from build123d import *

# Parameters (mm, degrees)
BOSS_EXTRUDE1_DEPTH = 135
SKETCH3_R           = 3.25
CUT_EXTRUDE2_DEPTH  = 10
SKETCH6_W           = 11
SKETCH6_H           = 36
CUT_EXTRUDE3_DEPTH  = 40
SKETCH7_W           = 55
SKETCH7_H           = 16.435142828
BOSS_EXTRUDE2_DEPTH = 35
CUT_EXTRUDE4_DEPTH  = 20
CUT_EXTRUDE5_DEPTH  = 20
SKETCH12_R          = 3.5
CUT_EXTRUDE6_DEPTH  = 10
CUT_EXTRUDE7_DEPTH  = 120
SKETCH14_W          = 10
SKETCH14_H          = 112.990035736
BOSS_EXTRUDE3_DEPTH = 9


with BuildPart() as part:
    # Sketch2 → Boss-Extrude1 (new body)
    with BuildSketch(Plane.XY):
        with BuildLine():
            Line((-7.403081865, 56.261800555), (-7.403081865, -78.738199445))
            ThreePointArc((-7.403081865, -78.738199445), (0.096918135, -86.238199445), (7.596918135, -78.738199445))
            Line((7.596918135, -78.738199445), (7.596918135, 56.261800555))
            ThreePointArc((7.596918135, 56.261800555), (0.096918135, 63.761800555), (-7.403081865, 56.261800555))
        make_face()
    extrude(amount=BOSS_EXTRUDE1_DEPTH)

    # Sketch3 → Cut-Extrude2 (cut)
    with BuildSketch(Plane(origin=(0, 0, 0), x_dir=(-1, 0, 0), z_dir=(0, 0, -1))):
        with Locations((-0.096918135, 54.761800555)):
            Circle(SKETCH3_R)
    extrude(amount=-CUT_EXTRUDE2_DEPTH, mode=Mode.SUBTRACT)

    # Sketch6 → Cut-Extrude3 (cut)
    with BuildSketch(Plane(origin=(0, 0, 0), x_dir=(-1, 0, 0), z_dir=(0, 0, -1))):
        with Locations((-0.096918135, -48.578199445)):
            Rectangle(SKETCH6_W, SKETCH6_H)
    extrude(amount=-CUT_EXTRUDE3_DEPTH, mode=Mode.SUBTRACT)

    # Sketch7 → Boss-Extrude2 (add)
    with BuildSketch(Plane.ZY.offset(7.403081865)):
        with Locations((67.5, -49.750557846)):
            Rectangle(SKETCH7_W, SKETCH7_H)
    extrude(amount=BOSS_EXTRUDE2_DEPTH)

    # Sketch10 → Cut-Extrude4 (cut)
    with BuildSketch(Plane(origin=(0, -41.532986432, 0), x_dir=(1, 0, 0), z_dir=(0, 1, 0))):
        with BuildLine():
            Line((-7.403081865, -40), (-42.403081865, -40))
            Line((-42.403081865, -40), (-42.403081865, -95))
            Line((-42.403081865, -95), (-7.403081865, -95))
            ThreePointArc((-7.403081865, -95), (-33.21161021, -67.5), (-7.403081865, -40))
        make_face()
    extrude(amount=-CUT_EXTRUDE4_DEPTH, mode=Mode.SUBTRACT)

    # Sketch11 → Cut-Extrude5 (cut)
    with BuildSketch(Plane(origin=(0, -41.532986432, 0), x_dir=(1, 0, 0), z_dir=(0, 1, 0))):
        with BuildLine():
            Line((-7.569996139, -52.041059143), (-7.569996139, -82.958940857))
            ThreePointArc((-7.569996139, -82.958940857), (-23.028936996, -67.5), (-7.569996139, -52.041059143))
        make_face()
    extrude(amount=-CUT_EXTRUDE5_DEPTH, mode=Mode.SUBTRACT)

    # Sketch12 → Cut-Extrude6 (cut)
    with BuildSketch(Plane.XY.offset(135)):
        with Locations((0.096918135, 54.761800555)):
            Circle(SKETCH12_R)
    extrude(amount=-CUT_EXTRUDE6_DEPTH, mode=Mode.SUBTRACT)

    # Sketch13 → Cut-Extrude7 (cut)
    with BuildSketch(Plane.XY.offset(135)):
        Polygon((4.403081865, 46.751836291), (-4.403081865, 46.751836291), (-4.403081865, -46.751836291), (-4.403081865, -66.238199445), (4.403081865, -66.238199445), (4.403081865, -46.751836291), align=None)
    extrude(amount=-CUT_EXTRUDE7_DEPTH, mode=Mode.SUBTRACT)

    # Sketch14 → Boss-Extrude3 (add)
    with BuildSketch(Plane.ZY.offset(-4.403081865)):
        with Locations((130, -9.743181577)):
            Rectangle(SKETCH14_W, SKETCH14_H)
    extrude(amount=BOSS_EXTRUDE3_DEPTH)


solid = part.part
Input: part model. Units: mm. Frame: model coordinates. A direction names the side the tool comes from. Give positions to 0.01 mm unless a question says otherwise; leave off trailing zeros. Loops run counter-clockwise (first coordinate to the right, second up) from the corner with the lowest first, then second, coordinate; pieces in that order, holes last. Notation, with made-up numbers: M 1.5,8 L 33.5,8 A30 ccw 33.5,33 Z; hole C -10,27.25 d6. An arc over 180 degrees is marked long. Use CSV: the item, a comma, the result in double quotes.
(1) Material intervals for L1, parallel to X at y = -18.5, z = 112; L2, parallel to Z at x = 0.5, y = -15; L3, parallel to Y at x = -4, z = 61.5, sorted ascending. Write a range as [from, to].
Outcome:
L1,"x = [-7.4, -4.4], [4.4, 7.6]"
L2,"z = [0, 15], [125, 135]"
L3,"y = [-85.02, -66.24], [46.75, 62.54]"
(2) Section A-A, the plane z = 67.5. Return loops of the section in (x, y), plus the area to 3 significant figures.
Outcome:
outline,"M -33.21,-57.97 L -23.03,-57.97 L -23.03,-41.53 L -33.21,-41.53 Z; M -7.57,-57.97 L -7.4,-57.97 L -7.4,-78.74 A7.5 ccw 7.6,-78.74 L 7.6,56.26 A7.5 ccw -7.4,56.26 L -7.4,-41.53 L -7.57,-41.53 Z; hole M -4.4,-66.24 L 4.4,-66.24 L 4.4,46.75 L -4.4,46.75 Z"
area,"1,380 mm²"
(3) Set-up query: faces 4 (the face through (-23.025, -49.636, 67.84)), 5 (the face through (4.403, -11, 71)), 6 (the face through (0, -66.238, 83)), 7 (the face through (-26, -57.968, 67)). Return all of +Z, -Z, +X, -X, +Y, -Y with unobstructed straight access to the full face (end or side cutting, diameter ignored); none if empty.
Outcome:
face 4,"+Y, -Y"
face 5,"none"
face 6,"-Z"
face 7,"+Z, -Z, -X, -Y"
(4) Section C-C, the plane y = -47. Return loops of the section in (x, z).
Outcome:
outline,"M -7.4,0 L -5.4,0 L -5.4,40 L -4.4,40 L -4.4,125 L 4.4,125 L 4.4,40 L 5.6,40 L 5.6,0 L 7.6,0 L 7.6,135 L -7.4,135 L -7.4,95 A27.56 ccw -7.4,40 Z; hole M -7.57,52.04 L -7.57,82.96 A15.46 ccw Z"
(5) Pull-direction query (Y, two-part tool) for faces 1 (the face through (-0.068, -86.236, 66.555)), 2 (the face through (7.597, -12, 67)), 3 (the face through (5, -48, 40)); classes: pulls with the +Y half, pulls with the -Y half, needs draft (parallel to the pull), parting line crosses it, or undercut.
Outcome:
face 1,"pulls with the -Y half"
face 2,"needs draft"
face 3,"undercut"
(6) Section D-D, the plane x = 1.5. Return loops of the section in (y, z).
Outcome:
outline,"M -86.11,0 L -66.58,0 L -66.58,40 L -66.24,40 L -66.24,125 L 46.75,125 L 46.75,15 L -30.58,15 L -30.58,0 L 51.83,0 L 51.83,10 L 57.69,10 L 57.69,0 L 63.63,0 L 63.63,135 L 57.97,135 L 57.97,125 L 51.56,125 L 51.56,135 L -86.11,135 Z"
(7) Pin query (flat end, axial travel): P1, Ø2, axis at y = -43, z = 112.5, coming from the -X side; P2, Ø10, axis at x = -14, y = -33.5, coming from the +Z side; P3, Ø13, axis at y = -52, z = 73, coming from the -X side; P4, Ø13, axis at x = -17.5, z = 75.5, coming from the +Y side. Return the tip coordinate at first contact, or that it passes through.
Outcome:
P1,"stops at x = -7.4"
P2,"passes through"
P3,"stops at x = -33.21"
P4,"stops at y = -41.53"
(8) Section B-B, the plane y = -22. Return loops of the section in (x, z), plus the area to 3 significant figures.
Outcome:
outline,"M -7.4,0 L 7.6,0 L 7.6,135 L -7.4,135 Z; hole M -4.4,15 L 4.4,15 L 4.4,125 L -4.4,125 Z"
area,"1,060 mm²"
